Work out the finished part from the listing and answer in its coordinate system (mm). Face numbers are marked on the shaded views. A direction names the side the tool comes from. Round coordinates to 2 decimals unless told otherwise and drop trailing zeros. Write each loop counter-clockwise with the first axis right and the second up, starting at its lowest first coordinate (ties: lowest second). Pieces come first, ordered by that corner, then holes. Notation, with made-up numbers: M 30.25,-9.75 L 87.25,-9.75 A34 ccw 87.25,20.25 Z; hole C 40.25,22 d10. An arc over 180 degrees is marked long. One line per item, written item: value. Start each with the question number.
Q1. The mould has two halves that part along X. Classify the marked faces 1, 2 and 3: released by +X, released by -X, zero draft, split by the parting line, or undercut.
Q2. Find section C-C (y = -24.5). Write down the section's boundary in (x, z), and give its area (3 significant figures).
Q3. A tool of negligible diameter and unlimited length cuts with its end or side. For the marked faces 4, 5 and 6, from which of +Z, -Z, +X, -X, +Y, -Y can it reach the whole face along a straight path? Write none if from no direction.
Q4. Given pin 1 Ø4.5 at (x, z) = (-12.37, -12.37) entering from +Y; pin 2 Ø13 at (x, z) = (-2, -2) entering from -Y; pin 3 Ø4 at (x, y) = (-10.5, -61) entering from -Z; pin 4 Ø4 at (y, z) = (-21, 5.5) entering from +X, each flat-ended and moving along its own axis, determine where each tip first touches the part or whether it passes through.
Q5. Find section D-D (z = 8). Write down the section's boundary in (x, y).
Q6. Consider probe 1 along Y at (x, z) = (0.5, 12.5); probe 2 along Y at (x, z) = (6, -17); probe 3 along Y at (x, z) = (-10, 19). Determine where each line is inside the solid, lowest interval first.
Q7. Find section B-B (x = 0). Write down the section's boundary in (y, z).
Q8. Find section A-A (z = 0). Write down the section's boundary in (x, y), and give its area (3 significant figures).
from build123d import *

# Parameters (mm, degrees)
SKETCH2_R          = 11
CUT_EXTRUDE1_DEPTH = 10
SKETCH3_W          = 5
SKETCH3_H          = 33.574223154
CUT_EXTRUDE2_DEPTH = 2
SKETCH4_R          = 2
CUT_EXTRUDE3_DEPTH = 9


with BuildPart() as part:
    # Sketch1 → Revolve1 (revolve)
    with BuildSketch(Plane.XY):
        Polygon((0, 0), (-13, 0), (-13, -2), (-22.5, -2), (-22.5, -46.9), (-21, -46.9), (-21, -50.9), (-22.25, -50.9), (-22.25, -113.4), (-6, -113.4), (-6, -118.4), (-2.5, -118.4), (-2.5, -128.4), (0, -128.4), align=None)
    revolve(axis=Axis((0, 0, 0), (0, -1, 0)))

    # Sketch2 → Cut-Extrude1 (cut)
    with BuildSketch(Plane(origin=(0, 0, 0), x_dir=(1, 0, 0), z_dir=(0, 1, 0))):
        Circle(SKETCH2_R)
    extrude(amount=-CUT_EXTRUDE1_DEPTH, mode=Mode.SUBTRACT)

    # Sketch3 → Cut-Extrude2 (cut)
    with BuildSketch(Plane(origin=(0, 0, 0), x_dir=(1, 0, 0), z_dir=(0, 1, 0))):
        with Locations((-14.5, 0)):
            Rectangle(SKETCH3_W, SKETCH3_H)
        with Locations((14.5, 0)):
            Rectangle(SKETCH3_W, SKETCH3_H)
    extrude(amount=-CUT_EXTRUDE2_DEPTH, mode=Mode.SUBTRACT)

    # Sketch4 → Cut-Extrude3 (cut)
    with BuildSketch(Plane(origin=(0, -2, 0), x_dir=(1, 0, 0), z_dir=(0, 1, 0))):
        with Locations((-12.374368671, 12.374368671)):
            Circle(SKETCH4_R)
        with Locations((12.374368671, 12.374368671)):
            Circle(SKETCH4_R)
        with Locations((12.374368671, -12.374368671)):
            Circle(SKETCH4_R)
        with Locations((-12.374368671, -12.374368671)):
            Circle(SKETCH4_R)
    extrude(amount=-CUT_EXTRUDE3_DEPTH, mode=Mode.SUBTRACT)


solid = part.part
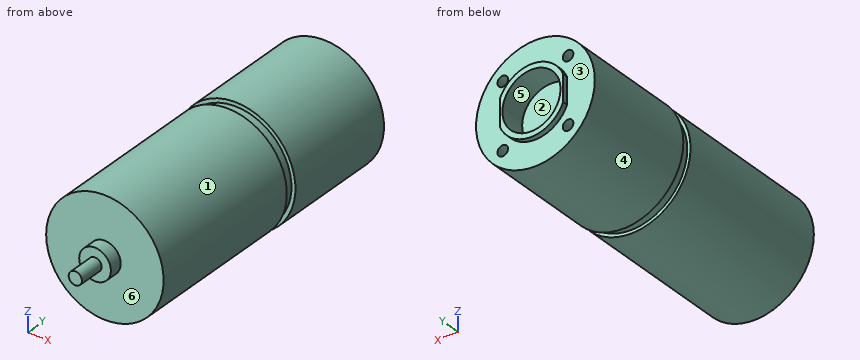
The answers:
1. face 1: split by the parting line
1. face 2: undercut
1. face 3: zero draft
2. outline: C 0,0 d45
2. area: 1,590 mm2
3. face 4: +Y, -Y
3. face 5: +Y
3. face 6: -Y
4. pin 1: y = -2
4. pin 2: y = -128.4
4. pin 3: z = -20.56
4. pin 4: x = 22.23
5. outline: M -21.03,-46.9 L -19.42,-46.9 L -19.42,-50.9 L -20.76,-50.9 L -20.76,-113.4 L 20.76,-113.4 L 20.76,-50.9 L 19.42,-50.9 L 19.42,-46.9 L 21.03,-46.9 L 21.03,-2 L 10.25,-2 L 10.25,0 L 7.55,0 L 7.55,-10 L -7.55,-10 L -7.55,0 L -10.25,0 L -10.25,-2 L -21.03,-2 Z
6. probe 1: -113.4 to 0
6. probe 2: -113.4 to -2
6. probe 3: -113.4 to -50.9, -46.9 to -2
7. outline: M -128.4,-2.5 L -118.4,-2.5 L -118.4,-6 L -113.4,-6 L -113.4,-22.25 L -50.9,-22.25 L -50.9,-21 L -46.9,-21 L -46.9,-22.5 L -2,-22.5 L -2,-13 L 0,-13 L 0,-11 L -10,-11 L -10,11 L 0,11 L 0,13 L -2,13 L -2,22.5 L -46.9,22.5 L -46.9,21 L -50.9,21 L -50.9,22.25 L -113.4,22.25 L -113.4,6 L -118.4,6 L -118.4,2.5 L -128.4,2.5 Z
8. outline: M -22.5,-46.9 L -21,-46.9 L -21,-50.9 L -22.25,-50.9 L -22.25,-113.4 L -6,-113.4 L -6,-118.4 L -2.5,-118.4 L -2.5,-128.4 L 2.5,-128.4 L 2.5,-118.4 L 6,-118.4 L 6,-113.4 L 22.25,-113.4 L 22.25,-50.9 L 21,-50.9 L 21,-46.9 L 22.5,-46.9 L 22.5,-2 L 12,-2 L 12,0 L 11,0 L 11,-10 L -11,-10 L -11,0 L -12,0 L -12,-2 L -22.5,-2 Z
8. area: 4,910 mm2
